Autodesk Inventor part; units mm, degrees
ref_plane "YZ Plane" through (0, 0, 0) normal (1, 0, 0) x (0, 1, 0)
ref_plane "XZ Plane" through (0, 0, 0) normal (0, 1, 0) x (-1, 0, 0)
ref_plane "XY Plane" through (0, 0, 0) normal (0, 0, 1) x (1, 0, 0)
sketch "Sketch1" plane through (0, 0, 0) normal (0, 0, 1) x (1, 0, 0)
  line L0 (0, 0) -> (0, 13.1) construction
  line L1 (4, 0) -> (4, 13.1)
  line L2 (4, 13.1) -> (8, 13.1)
  line L3 (8, 13.1) -> (8, 3.1)
  line L4 (8, 3.1) -> (16, 3.1)
  line L5 (16, 3.1) -> (16, 0)
  line L6 (16, 0) -> (4, 0)
  point P0 (8, 8.1)
  point P1 (8, 8.1)
  dimension "d0" = 13.1
  dimension "d1" = 10
  dimension "d2" = 3.1
  dimension "d3" = 32
  dimension "d4" = 16
  dimension "d5" = 8
revolve "Revolution1" add sketch "Sketch1" angle 360 about axis through (0, 0, 0) along (0, 1, 0)
sketch "Sketch2" plane through (0, 0, 0) normal (0, -1, 0) x (1, 0, 0)
  circle A0 centre (11.95, 0) radius 2
  line L0 (13.95, 0) -> (16, 0) construction
  circle A1 centre (0, 0) radius 16 construction
  dimension "d7" = 4
  dimension "d8" = 2.05
extrude "MountHole" cut sketch "Sketch2" against normal through all
pattern_circular "Circular Pattern1" count 4 over 360 about axis through (0, 6.55, 0) along (0, -1, 0) of "MountHole"
equation "\"d0\" = flangeCoupling_height"
equation "\"d1\" = flangeCoupling_collarHeight"
equation "\"d2\" = flangeCoupling_flangeHeight"
equation "\"d3\" = flangeCoupling_flangeDiameter"
equation "\"d4\" = flangeCoupling_collarOuterDiameter"
equation "\"d5\" = flangeCoupling_innerDiameter"
equation "\"d7\" = flangeCoupling_mountHoleDiameter + gap"
equation "\"d8\" = flangeCoupling_mountHoleEdgeToEdge"
equation "\"gap\" = 0.1"
equation "\"airgap\" = 0.4"
equation "\"wallgap\" = 2"
equation "\"driveMagnet_height\" = 5"
equation "\"halbachMagnet_height\" = 3"
equation "\"rotorBandBolt_diameter\" = 2"
equation "\"rotorBandBolt_headDiameter\" = 3.98"
equation "\"rotorBandBolt_headHeight\" = 2"
equation "\"rotorBandHexNut_sideToSide\" = 4"
equation "\"rotorBandHexNut_height\" = 1.2"
equation "\"rotorBandSquareNut_sideLength\" = 4"
equation "\"rotorBandSquareNut_height\" = 1.2"
equation "\"sensorMagnet_diameter\" = 5"
equation "\"sensorMagnet_height\" = 2.66667"
equation "\"rotorRadius\" = 2 * gap + driveMagnet_centerSpacingRadius + driveMagnet_length + wallgap"
equation "\"rotor_mountingLipHeight\" = 0.5 * statorThickness"
equation "\"shaftDiameter\" = 8"
equation "\"flangeBearing_innerDiameter\" = shaftDiameter"
equation "\"flangeBearing_outerDiameter\" = 16"
equation "\"flangeBearing_flangeDiameter\" = 18"
equation "\"flangeBearing_height\" = 5"
equation "\"flangeBearing_flangeHeight\" = 1"
equation "\"statorThickness\" = coilThickness + 2 * wallgap"
equation "\"rotorBandThickness\" = wallgap + rotorBandBolt_headHeight + gap"
equation "\"flangeCoupling_innerDiameter\" = shaftDiameter"
equation "\"flangeCoupling_collarOuterDiameter\" = 16"
equation "\"flangeCoupling_flangeDiameter\" = 32"
equation "\"flangeCoupling_collarHeight\" = 10"
equation "\"flangeCoupling_flangeHeight\" = 3.1"
equation "\"flangeCoupling_flangeHoleDiameter\" = 3.9"
equation "\"flangeCoupling_flangeHoleEdgeToEdge\" = 2.05"
equation "\"flangeCoupling_height\" = flangeCoupling_collarHeight + flangeCoupling_flangeHeight"
equation "\"flangeCoupling_mountHoleDiameter\" = 3.9"
equation "\"flangeCoupling_mountHoleEdgeToEdge\" = 2.05"
equation "\"statorRadius\" = driveMagnet_length + driveMagnet_centerSpacingRadius + 2 * gap"
equation "\"coilThickness\" = 12"
equation "\"statorMountBolt_diameter\" = 4"
equation "\"statorMountBolt_headDiameter\" = 7"
equation "\"statorMountBolt_headHeight\" = 4"
equation "\"statorMountBolt_shaftLength\" = coilThickness + flangeCoupling_flangeHeight + wallgap"
equation "\"statorMountHexNut_height\" = 4"
equation "\"statorMountHexNut_sideToSide\" = 8"
equation "\"sensorMagnet_ringRadius\" = 0.5 * driveMagnet_centerSpacingRadius + 2 * wallgap"
equation "\"coil_percentCoverage\" = 0.6"
equation "\"statorSpokeDegrees\" = 4deg"
equation "\"coil_bulge\" = 3"
equation "\"statorCoilBolt_shaftLength\" = coilThickness"
equation "\"statorCoilHexNut_height\" = 1.2"
equation "\"statorCoilBolt_headHeight\" = 2"
equation "\"statorCoilBolt_diameter\" = 2"
equation "\"statorCoilBolt_headDiameter\" = 3.98"
equation "\"statorCoilHexNut_sideToSide\" = 4"
equation "\"magnetWire_outerDiameter\" = 0.8128"
equation "\"printingLayerHeight\" = 0.2"
equation "\"circuitBoard_height\" = 1.6"
equation "\"hallEffectSensor_width\" = 1.6"
equation "\"hallEffectSensor_length\" = 3"
equation "\"hallEffectSensor_height\" = 1.1"
equation "\"hallEffectSensor_pinLength\" = 0.6"
equation "\"circuitboardMountHexNut_height\" = 1.2"
equation "\"circuitboardMountHexNut_sideToSide\" = 4"
equation "\"circuitboardMountBolt_headHeight\" = 2"
equation "\"circuitboardMountBolt_shaftLength\" = coilThickness"
equation "\"circuitboardMountBolt_diameter\" = 2"
equation "\"circuitboardMountBolt_headDiameter\" = 3.98"
equation "\"statorShellBolt_headDiameter\" = 5.68"
equation "\"statorShellHexNut_height\" = 2.3"
equation "\"statorShellBolt_shaftLength\" = statorThickness - statorShellBolt_countersinkDepth"
equation "\"statorShellBolt_headHeight\" = 3"
equation "\"statorShellHexNut_sideToSide\" = 5.3"
equation "\"statorShellBolt_diameter\" = 3"
properties part number "FlangeCoupling" material "Steel, Mild"
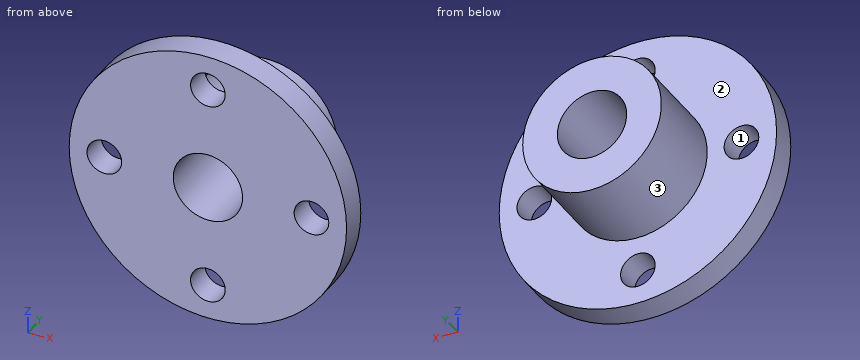
Work out the finished part from the listing and answer in its coordinate system (mm). Face numbers are marked on the shaded views. Round coordinates to 2 decimals unless told otherwise and drop trailing zeros. Loops run counter-clockwise (first coordinate to the right, second up) from the corner with the lowest first, then second, coordinate; pieces in that order, holes last. Notation, with made-up numbers: M -35,-36.5 L -29,-36.5 A16 cw -29,-31.5 Z; hole C 47,87.5 d9. An arc over 180 degrees is marked long. Use CSV: the item, a comma, the result in double quotes.
Q1. Section B-B, the plane x = 0 is taken. Determine the outline of the cut face in (y, z), then the cut area to 3 significant figures.
Determined:
outline,"M 0,-16 L 3.1,-16 L 3.1,-13.95 L 0,-13.95 Z; M 0,-9.95 L 3.1,-9.95 L 3.1,-8 L 13.1,-8 L 13.1,-4 L 0,-4 Z; M 0,4 L 13.1,4 L 13.1,8 L 3.1,8 L 3.1,9.95 L 0,9.95 Z; M 0,13.95 L 3.1,13.95 L 3.1,16 L 0,16 Z"
area,"130 mm2"
Q2. Each of these flat-tipped pins is pushed along its axis until it touches: pin 1 (2.5 mm diameter, centred on x = 11.95, z = 0, fed in from +Y); pin 2 (1.5 mm diameter, centred on y = 2, z = 4.5, fed in from -X); pin 3 (1 mm diameter, centred on x = 3.5, y = 5, fed in from -Z); pin 4 (1.5 mm diameter, centred on x = 3, y = 8.5, fed in from -Z). Where does it stop, or does it pass through?
Determined:
pin 1,"through"
pin 2,"x = -15.55"
pin 3,"z = -7.42"
pin 4,"z = -7.68"
Q3. The mould has two halves that part along Z. Classify the marked faces 1, 2 and 3: pulls with the +Z half, pulls with the -Z half, needs draft (parallel to the pull), parting line crosses it, or undercut.
Determined:
face 1,"undercut"
face 2,"needs draft"
face 3,"parting line crosses it"
Q4. Section A-A, the plane z = 0 is taken. Determine the outline of the cut face in (x, y), then the cut area to 3 significant figures.
Determined:
outline,"M -16,0 L -13.95,0 L -13.95,3.1 L -16,3.1 Z; M -9.95,0 L -4,0 L -4,13.1 L -8,13.1 L -8,3.1 L -9.95,3.1 Z; M 4,0 L 9.95,0 L 9.95,3.1 L 8,3.1 L 8,13.1 L 4,13.1 Z; M 13.95,0 L 16,0 L 16,3.1 L 13.95,3.1 Z"
area,"130 mm2"
Q5. Section C-C, the plane z = -11 is taken. Determine the outline of the cut face in (x, y), then the cut area to 3 significant figures.
Determined:
outline,"M -11.62,0 L -1.76,0 L -1.76,3.1 L -11.62,3.1 Z; M 1.76,0 L 11.62,0 L 11.62,3.1 L 1.76,3.1 Z"
area,"61.1 mm2"
Q6. Consider L1, parallel to Z at x = 0, y = 8.5; L2, parallel to Y at x = -8, z = -7.5. Determine where each line is inside the solid, lowest interval first.
Determined:
L1,"-8 to -4, 4 to 8"
L2,"0 to 3.1"
Q7. Section D-D, the plane x = -12.5 is taken. Determine the outline of the cut face in (y, z).
Determined:
outline,"M 0,-9.99 L 3.1,-9.99 L 3.1,-1.92 L 0,-1.92 Z; M 0,1.92 L 3.1,1.92 L 3.1,9.99 L 0,9.99 Z"
